Design review of the part built by this model. Coordinates are the model's own, in mm. A direction names the side the tool comes from. Give positions to 0.01 mm unless a question says otherwise; leave off trailing zeros. Write each loop counter-clockwise with the first axis right and the second up, starting at its lowest first coordinate (ties: lowest second). Pieces come first, ordered by that corner, then holes. Notation, with made-up numbers: M 48.25,22 L 73.25,22 A12 ccw 73.25,42 Z; hole C -25,60.5 d6. An arc over 180 degrees is marked long. Use one line per item in the form item = value. Start each with the question number.
from build123d import *

# Parameters (mm, degrees)
PAD_DEPTH       = 19.5
SKETCH001_R     = 1.6
POCKET_DEPTH    = 19.501
SKETCH002_R     = 1.6
POCKET001_DEPTH = 12.001
POCKET002_DEPTH = 2.4
POCKET003_DEPTH = 2.4
POCKET004_DEPTH = 2.4


with BuildPart() as part:
    # Sketch → Pad (new body)
    with BuildSketch(Plane.XY):
        with BuildLine():
            ThreePointArc((6, 7.5), (0, 13.5), (-6, 7.5))
            Line((-6, 7.5), (-6, -7.5))
            Line((-6, -7.5), (6, -7.5))
            Line((6, -7.5), (6, 7.5))
        make_face()
    extrude(amount=PAD_DEPTH)

    # Sketch001 (on Face5 of Pad) → Pocket (cut, through all)
    with BuildSketch(Plane(origin=(0, 0, 0), x_dir=(1, 0, 0), z_dir=(0, 0, -1))):
        with Locations((0, -7.5)):
            Circle(SKETCH001_R)
    extrude(amount=-POCKET_DEPTH, mode=Mode.SUBTRACT)

    # Sketch002 (on Face3 of Pocket) → Pocket001 (cut, through all)
    with BuildSketch(Plane(origin=(-6, 0, 0), x_dir=(0, -1, 0), z_dir=(-1, 0, 0))):
        with Locations((3, 14.625)):
            Circle(SKETCH002_R)
        with Locations((3, 4.875)):
            Circle(SKETCH002_R)
    extrude(amount=-POCKET001_DEPTH, mode=Mode.SUBTRACT)

    # Sketch003 (on Face3 of Pocket001) → Pocket002 (cut)
    with BuildSketch(Plane(origin=(-6, 0, 0), x_dir=(0, -1, 0), z_dir=(-1, 0, 0))):
        Polygon((3, 17.858162), (0.2, 16.241581), (0.2, 13.008419), (3, 11.391838), (5.8, 13.008419), (5.8, 16.241581), align=None)
        Polygon((3, 8.108162), (0.2, 6.491581), (0.2, 3.258419), (3, 1.641838), (5.8, 3.258419), (5.8, 6.491581), align=None)
    extrude(amount=-POCKET002_DEPTH, mode=Mode.SUBTRACT)

    # Sketch004 (on Face4 of Pocket002) → Pocket003 (cut)
    with BuildSketch(Plane(origin=(0, 0, 0), x_dir=(1, 0, 0), z_dir=(0, 0, -1))):
        Polygon((2.8, -9.116581), (2.8, -5.883419), (0, -4.266838), (-2.8, -5.883419), (-2.8, -9.116581), (0, -10.733162), align=None)
    extrude(amount=-POCKET003_DEPTH, mode=Mode.SUBTRACT)

    # Sketch005 (on Face5 of Pocket003) → Pocket004 (cut)
    with BuildSketch(Plane.XY.offset(19.5)):
        Polygon((2.8, 9.116581), (0, 10.733162), (-2.8, 9.116581), (-2.8, 5.883419), (0, 4.266838), (2.8, 5.883419), align=None)
    extrude(amount=-POCKET004_DEPTH, mode=Mode.SUBTRACT)


solid = part.part
1. For faces 4 (the flat face through (-1, 9, 2.4)), 5 (the flat face through (-1.42, 5.086, 18.317)), 6 (the flat face through (-5, -0.2, 5)), list the 3-axis set-ups (+Z, -Z, +X, -X, +Y, -Y) from which the entire face can be reached by the end or side of a thin tool; tool diameter is ignored.
2. We need section A-A (z = 18.5). State the section outline as (x, y) points, and give its area (3 significant figures).
3. Clearance check with flat-ended pins moving along their axes: pin 1 Ø4 at (y, z) = (-3, 14.625) entering from -X; pin 2 Ø1.2 at (x, z) = (-4.5, 5) entering from +Y; pin 3 Ø4.5 at (y, z) = (-2.5, 4) entering from -X; pin 4 Ø2 at (x, y) = (-1.5, 8) entering from +Z. State where each tip first meets the part, or that it passes through.
4. We need section C-C (z = 9.25). State the section outline as (x, y) points, and give its area (3 significant figures).
5. We need section B-B (y = -3.5). State the section outline as (x, z) points, and give its area (3 significant figures).
6. Draft analysis for pull direction X (two halves, no side actions). For faces 1 (the flat face through (-3.6, -2, 3)), 2 (the flat face through (-4.82, -1.58, 2.46)), 3 (the cylindrical face through (-0.35, 9.06, 9.65)), state which applies: pulls with the +X half, pulls with the -X half, needs draft (parallel to the pull), parting line crosses it, or undercut.
7. To check wall thickness, follow L1, parallel to Z at x = 3.5, y = -3 (3 decimals); L2, parallel to Z at x = -5, y = -3.25; L3, parallel to X at y = 7.5, z = 3.5. State the ranges of each line that lie inside material, in increasing order.
8. We need section D-D (y = 11.5). State the section outline as (x, z) points.
Answer block:
q1.face_4 = -Z
q1.face_5 = +Z
q1.face_6 = -X
q2.outline = M -6,-7.5 L 6,-7.5 L 6,7.5 A6 ccw -6,7.5 Z; hole M -2.8,5.88 L 0,4.27 L 2.8,5.88 L 2.8,9.12 L 0,10.73 L -2.8,9.12 Z
q2.area = 209 mm^2
q3.pin_1 = -3.6
q3.pin_2 = 12.06
q3.pin_3 = -6
q3.pin_4 = 17.1
q4.outline = M -6,-7.5 L 6,-7.5 L 6,7.5 A6 ccw -6,7.5 Z; hole C 0,7.5 d3.2
q4.area = 229 mm^2
q5.outline = M -6,0 L 6,0 L 6,3.36 L -3.6,3.36 L -3.6,1.93 L -6,1.93 Z; M -6,7.82 L -3.6,7.82 L -3.6,6.39 L 6,6.39 L 6,13.11 L -3.6,13.11 L -3.6,11.68 L -6,11.68 Z; M -6,17.57 L -3.6,17.57 L -3.6,16.14 L 6,16.14 L 6,19.5 L -6,19.5 Z
q5.area = 147 mm^2
q6.face_1 = pulls with the -X half
q6.face_2 = needs draft
q6.face_3 = undercut
q7.L1 = 0 to 3.275, 6.475 to 13.025, 16.225 to 19.5
q7.L2 = 0 to 1.79, 7.96 to 11.54, 17.71 to 19.5
q7.L3 = -6 to -1.6, 1.6 to 6
q8.outline = M -4.47,0 L 4.47,0 L 4.47,19.5 L -4.47,19.5 Z
